CAD build for the part. Positions are in the model's coordinates, mm. A direction names the side the tool comes from. Coordinates: 2 decimals unless noted, no trailing zeros. Write each loop counter-clockwise with the first axis right and the second up, starting at its lowest first coordinate (ties: lowest second). Pieces come first, ordered by that corner, then holes. Notation, with made-up numbers: (45, -14.75) - (82, -14.75) arc R35 cw to (82, 20.25) - close; hole circle Ø1 at (19, 10.5). An arc over 180 degrees is marked (long way). Answer in a Markdown table with one row per item. Add a question column.
Q1. Band-saw the part on D-D (y = 2.35). List the corners of the cut face in (x, z).
Q2. 3-axis set-ups, long thin cutter, end or side, ignore diameter. For faces 5 (the flat face through (-16, 2, -6)), 6 (the flat face through (-10, 2, 2.1)): which of +Z, -Z, +X, -X, +Y, -Y reach the whole face in a straight line?
Q3. Pin check, flat tips, straight feed: pin 1 (2 mm diameter, centred on y = 1.5, z = -8, fed in from +X); pin 2 (1 mm diameter, centred on y = 3.5, z = -4, fed in from +X). Stop position of each tip, or through.
Q4. Band-saw the part on C-C (x = -11.5). List the corners of the cut face in (y, z), and give its area (3 significant figures).
Q5. Band-saw the part on B-B (x = 8.8). List the corners of the cut face in (y, z), and give its area (3 significant figures).
Q6. Band-saw the part on A-A (z = 5.75). List the corners of the cut face in (x, y), and give its area (3 significant figures).
Q7. Drill centre lines: line 1 along X through (y, z) = (3.3, 1); line 2 along Z through (x, y) = (-8.8, 1.45); line 3 along Z through (x, y) = (12, 2.7). Where is each one in solid material? Low to high. Write a range as from..to.
Q8. Two-plate mould, pull along Z, no slides. Class faces 1 (the flat face through (-20, 2, 0)), 2 (the flat face through (0, 2, -10)), 3 (the flat face through (16, 2, 6)), 4 (the flat face through (10, 2, 2.1)): +Z half, -Z half, draft (parallel to the pull), parting line (faces both ways), or undercut.
```python
from build123d import *

# Parameters (mm, degrees)
BOSS_EXTRUDE1_DEPTH = 4
SKETCH2_W           = 8.2
SKETCH2_H           = 4.2
CUT_EXTRUDE1_DEPTH  = 4
SKETCH3_R           = 1.75
CUT_EXTRUDE2_DEPTH  = 4


with BuildPart() as part:
    # Sketch1 → Boss-Extrude1 (new body)
    with BuildSketch(Plane(origin=(0, 0, 0), x_dir=(1, 0, 0), z_dir=(0, 1, 0))):
        Polygon((12, -10), (-12, -10), (-20, -2), (-20, 2), (-12, 10), (12, 10), (20, 2), (20, -2), align=None)
    extrude(amount=BOSS_EXTRUDE1_DEPTH)

    # Sketch2 → Cut-Extrude1 (cut)
    with BuildSketch(Plane(origin=(0, 4, 0), x_dir=(1, 0, 0), z_dir=(0, 1, 0))):
        with Locations((9.9, 0)):
            Rectangle(SKETCH2_W, SKETCH2_H)
        with Locations((-9.9, 0)):
            Rectangle(SKETCH2_W, SKETCH2_H)
    extrude(amount=-CUT_EXTRUDE1_DEPTH, mode=Mode.SUBTRACT)

    # Sketch3 → Cut-Extrude2 (cut)
    with BuildSketch(Plane(origin=(0, 4, 0), x_dir=(1, 0, 0), z_dir=(0, 1, 0))):
        with Locations((-8.8, -5.75)):
            Circle(SKETCH3_R)
        with Locations((8.8, -5.75)):
            Circle(SKETCH3_R)
    extrude(amount=-CUT_EXTRUDE2_DEPTH, mode=Mode.SUBTRACT)


solid = part.part
```
Checked values:
| question | item | result |
|---|---|---|
| 1 | outline | (-20, -2) - (-12, -10) - (12, -10) - (20, -2) - (20, 2) - (12, 10) - (-12, 10) - (-20, 2) - close; hole (-14, -2.1) - (-5.8, -2.1) - (-5.8, 2.1) - (-14, 2.1) - close; hole circle Ø3.5 at (-8.8, 5.75); hole (5.8, -2.1) - (14, -2.1) - (14, 2.1) - (5.8, 2.1) - close; hole circle Ø3.5 at (8.8, 5.75) |
| 2 | face 5 | -Z, -X, +Y, -Y |
| 2 | face 6 | +Y, -Y |
| 3 | pin 1 | stops at x = 15 |
| 3 | pin 2 | stops at x = 18.5 |
| 4 | outline | (0, -10) - (4, -10) - (4, -2.1) - (0, -2.1) - close; (0, 2.1) - (4, 2.1) - (4, 10) - (0, 10) - close |
| 4 | area | 63.2 mm² |
| 5 | outline | (0, -10) - (4, -10) - (4, -2.1) - (0, -2.1) - close; (0, 2.1) - (4, 2.1) - (4, 4) - (0, 4) - close; (0, 7.5) - (4, 7.5) - (4, 10) - (0, 10) - close |
| 5 | area | 49.2 mm² |
| 6 | outline | (-16.25, 0) - (-10.55, 0) - (-10.55, 4) - (-16.25, 4) - close; (-7.05, 0) - (7.05, 0) - (7.05, 4) - (-7.05, 4) - close; (10.55, 0) - (16.25, 0) - (16.25, 4) - (10.55, 4) - close |
| 6 | area | 102 mm² |
| 7 | line 1 | x = -20..-14, -5.8..5.8, 14..20 |
| 7 | line 2 | z = -10..-2.1, 2.1..4, 7.5..10 |
| 7 | line 3 | z = -10..-2.1, 2.1..10 |
| 8 | face 1 | draft |
| 8 | face 2 | -Z half |
| 8 | face 3 | +Z half |
| 8 | face 4 | undercut |
